Geometry: final body of the model. Coordinates: model frame, mm. A direction names the side the tool comes from. Give positions to 0.01 mm unless a question says otherwise; leave off trailing zeros. Write each loop counter-clockwise with the first axis right and the second up, starting at its lowest first coordinate (ties: lowest second). Pieces come first, ordered by that corner, then holes.
```python
from build123d import *

# Parameters (mm, degrees)
SKETCH1_W              = 2
SKETCH1_H              = 0.3
BOSS_EXTRUDE1_DEPTH    = 50
SKETCH1_H_2            = 0.6
BOSS_EXTRUDE1_2_DEPTH  = 50
SKETCH1_H_3            = 0.9
BOSS_EXTRUDE1_3_DEPTH  = 50
SKETCH1_H_4            = 1.2
BOSS_EXTRUDE1_4_DEPTH  = 50
SKETCH1_H_5            = 1.5
BOSS_EXTRUDE1_5_DEPTH  = 50
SKETCH1_H_6            = 1.8
BOSS_EXTRUDE1_6_DEPTH  = 50
SKETCH1_H_7            = 2.1
BOSS_EXTRUDE1_7_DEPTH  = 50
SKETCH1_H_8            = 2.4
BOSS_EXTRUDE1_8_DEPTH  = 50
SKETCH1_H_9            = 2.7
BOSS_EXTRUDE1_9_DEPTH  = 50
SKETCH1_H_10           = 3
BOSS_EXTRUDE1_10_DEPTH = 50
SKETCH1_H_11           = 3.3
BOSS_EXTRUDE1_11_DEPTH = 50
SKETCH1_H_12           = 3.6
BOSS_EXTRUDE1_12_DEPTH = 50
BOSS_EXTRUDE2_DEPTH    = 2


with BuildPart() as part:
    # Sketch1 → Boss-Extrude1 (new body)
    with BuildSketch(Plane.XY):
        with Locations((1, 0.15)):
            Rectangle(SKETCH1_W, SKETCH1_H)
    extrude(amount=BOSS_EXTRUDE1_DEPTH)



with BuildPart() as body_2:
    # Sketch1 → Boss-Extrude1 2 (new body)
    with BuildSketch(Plane.XY):
        with Locations((3.5, 0.3)):
            Rectangle(SKETCH1_W, SKETCH1_H_2)
    extrude(amount=BOSS_EXTRUDE1_2_DEPTH)


with BuildPart() as body_3:
    # Sketch1 → Boss-Extrude1 3 (new body)
    with BuildSketch(Plane.XY):
        with Locations((6, 0.45)):
            Rectangle(SKETCH1_W, SKETCH1_H_3)
    extrude(amount=BOSS_EXTRUDE1_3_DEPTH)


with BuildPart() as body_4:
    # Sketch1 → Boss-Extrude1 4 (new body)
    with BuildSketch(Plane.XY):
        with Locations((8.5, 0.6)):
            Rectangle(SKETCH1_W, SKETCH1_H_4)
    extrude(amount=BOSS_EXTRUDE1_4_DEPTH)


with BuildPart() as body_5:
    # Sketch1 → Boss-Extrude1 5 (new body)
    with BuildSketch(Plane.XY):
        with Locations((11, 0.75)):
            Rectangle(SKETCH1_W, SKETCH1_H_5)
    extrude(amount=BOSS_EXTRUDE1_5_DEPTH)


with BuildPart() as body_6:
    # Sketch1 → Boss-Extrude1 6 (new body)
    with BuildSketch(Plane.XY):
        with Locations((13.5, 0.9)):
            Rectangle(SKETCH1_W, SKETCH1_H_6)
    extrude(amount=BOSS_EXTRUDE1_6_DEPTH)


with BuildPart() as body_7:
    # Sketch1 → Boss-Extrude1 7 (new body)
    with BuildSketch(Plane.XY):
        with Locations((16, 1.05)):
            Rectangle(SKETCH1_W, SKETCH1_H_7)
    extrude(amount=BOSS_EXTRUDE1_7_DEPTH)


with BuildPart() as body_8:
    # Sketch1 → Boss-Extrude1 8 (new body)
    with BuildSketch(Plane.XY):
        with Locations((18.5, 1.2)):
            Rectangle(SKETCH1_W, SKETCH1_H_8)
    extrude(amount=BOSS_EXTRUDE1_8_DEPTH)


with BuildPart() as body_9:
    # Sketch1 → Boss-Extrude1 9 (new body)
    with BuildSketch(Plane.XY):
        with Locations((21, 1.35)):
            Rectangle(SKETCH1_W, SKETCH1_H_9)
    extrude(amount=BOSS_EXTRUDE1_9_DEPTH)


with BuildPart() as body_10:
    # Sketch1 → Boss-Extrude1 10 (new body)
    with BuildSketch(Plane.XY):
        with Locations((23.5, 1.5)):
            Rectangle(SKETCH1_W, SKETCH1_H_10)
    extrude(amount=BOSS_EXTRUDE1_10_DEPTH)


with BuildPart() as body_11:
    # Sketch1 → Boss-Extrude1 11 (new body)
    with BuildSketch(Plane.XY):
        with Locations((26, 1.65)):
            Rectangle(SKETCH1_W, SKETCH1_H_11)
    extrude(amount=BOSS_EXTRUDE1_11_DEPTH)


with BuildPart() as body_12:
    # Sketch1 → Boss-Extrude1 12 (new body)
    with BuildSketch(Plane.XY):
        with Locations((28.5, 1.8)):
            Rectangle(SKETCH1_W, SKETCH1_H_12)
    extrude(amount=BOSS_EXTRUDE1_12_DEPTH)


with BuildPart() as part_1:
    add(part.part)

    add(body_2.part)  # Boss-Extrude2 merges body 2

    add(body_3.part)  # Boss-Extrude2 merges body 3

    add(body_4.part)  # Boss-Extrude2 merges body 4

    add(body_5.part)  # Boss-Extrude2 merges body 5

    add(body_6.part)  # Boss-Extrude2 merges body 6

    add(body_7.part)  # Boss-Extrude2 merges body 7

    add(body_8.part)  # Boss-Extrude2 merges body 8

    add(body_9.part)  # Boss-Extrude2 merges body 9

    add(body_10.part)  # Boss-Extrude2 merges body 10

    add(body_11.part)  # Boss-Extrude2 merges body 11

    add(body_12.part)  # Boss-Extrude2 merges body 12
    # Sketch2 → Boss-Extrude2 (add)
    with BuildSketch(Plane.XY.offset(50)):
        Polygon((0, 0), (29.5, 0), (29.5, 3.6), (27.5, 3.6), (0, 0.3), align=None)
    extrude(amount=BOSS_EXTRUDE2_DEPTH)


solid = part_1.part
```
Item 1: Section C-C, the plane x = 15.75. Return the cut outline in (y, z), plus the area to 3 significant figures.
Found:
outline: (0, 0) - (2.1, 0) - (2.1, 50) - (2.19, 50) - (2.19, 52) - (0, 52) - close
area: 109 mm2
Item 2: Pull-direction query (X, two-part tool) for faces 1 (the face through (22, 1, 25)), 2 (the face through (18, 2.4, 25)); classes: +X half, -X half, draft (parallel to the pull), parting line (faces both ways), or undercut.
Found:
face 1: undercut
face 2: draft
Item 3: Reachability of faces 3 (the face through (16, 1, 0)), 4 (the face through (1, 0.3, 25)), 5 (the face through (12, 1, 25)) from +Z, -Z, +X, -X, +Y, -Y: full face, straight path, thin tool, end or side. Return the list, or none.
Found:
face 3: -Z, +X, -X, +Y, -Y
face 4: -Z, -X, +Y
face 5: -Z, +Y, -Y
Item 4: Line query: L1, parallel to X at y = 2.3, z = 26; L2, parallel to X at y = 2.75, z = 16.5; L3, parallel to X at y = 3.05, z = 4.5. Output: solid intervals per line, ascending.
Found:
L1: x = 17.5 to 19.5, 20 to 22, 22.5 to 24.5, 25 to 27, 27.5 to 29.5
L2: x = 22.5 to 24.5, 25 to 27, 27.5 to 29.5
L3: x = 25 to 27, 27.5 to 29.5
Item 5: Section B-B, the plane z = 6. State how many separate pieces and enclosed holes the cut face has, plus the area to 3 significant figures.
Found:
separate pieces: 12
enclosed holes: 0
area: 46.8 mm2
Item 6: Pin query (flat end, axial travel): pin 1 Ø0.6 at (x, z) = (3.5, 36) entering from +Y; pin 2 Ø2 at (x, z) = (23.5, 28) entering from +Y; pin 3 Ø1.5 at (x, z) = (12.5, 7) entering from +Y. Return the tip coordinate at first contact, or that it passes through.
Found:
pin 1: stops at y = 0.6
pin 2: stops at y = 3
pin 3: stops at y = 1.8
Item 7: Section A-A, the plane x = 5.5. Return the cut outline in (y, z), plus the area to 3 significant figures.
Found:
outline: (0, 0) - (0.9, 0) - (0.9, 50) - (0.96, 50) - (0.96, 52) - (0, 52) - close
area: 46.9 mm2
